The figure shows three views and two pictorial views of one solid part (mm, origin at its lowest corner). Answer the questions. A direction names the side the tool comes from. Coordinates: 2 decimals unless noted, no trailing zeros. Order: outer loops, then holes, each group sorted by start corner. A loop starts at its lowest first (then second) coordinate and runs counter-clockwise, first axis right, second up. Notation, with made-up numbers: (10.5, 67.25) - (53.5, 67.25) arc R29 cw to (53.5, 91.25) - close; hole circle Ø11 at (-6, 21.25). An arc over 180 degrees is marked (long way). Use one line per item in the form item = value.
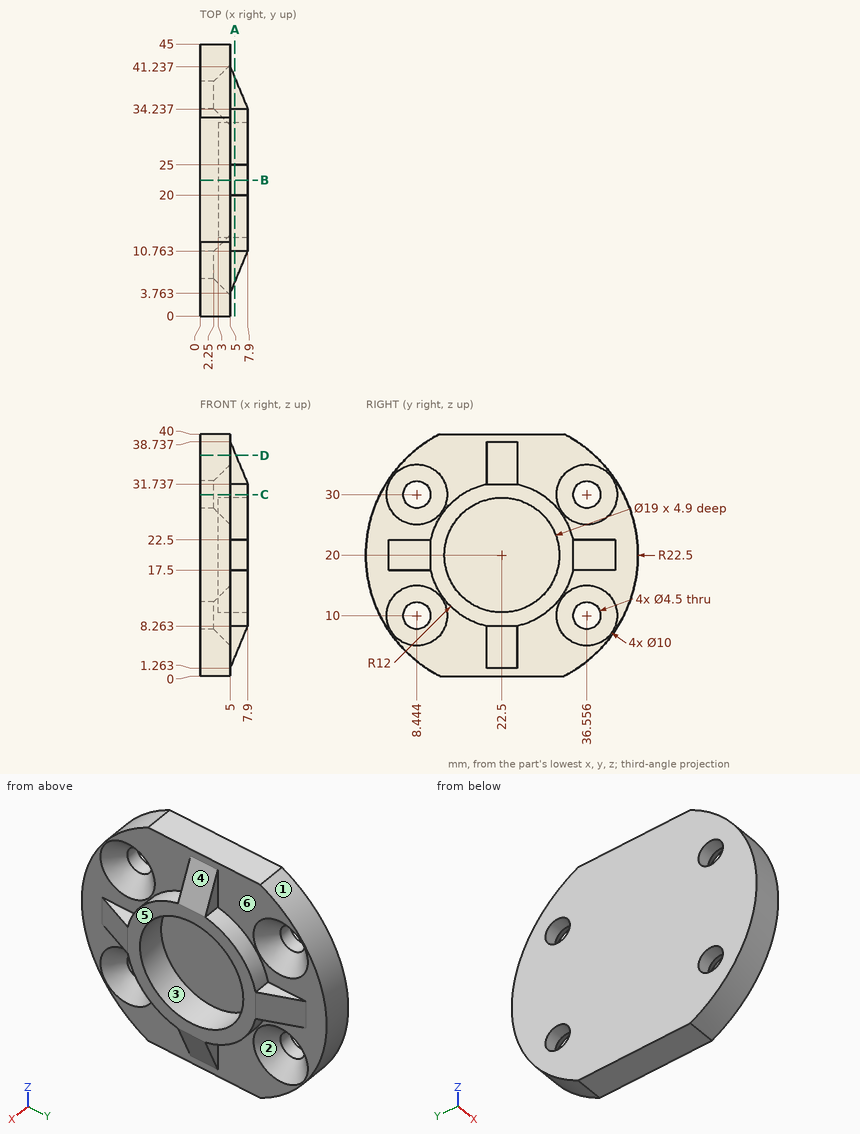
(1) The mould has two halves that part along Y. Classify the marked faces 1, 2, 3 and 4: +Y half, -Y half, draft (parallel to the pull), parting line (faces both ways), or undercut.
Answer list:
face_1 = +Y half
face_2 = undercut
face_3 = undercut
face_4 = draft
(2) Section A-A, the plane x = 5.75 is taken. Write down the section's boundary in (y, z), then the cut area to 3 significant figures.
Answer list:
outline = (5.57, 17.5) - (10.76, 17.5) arc R12 ccw to (20, 8.26) - (20, 3.07) - (25, 3.07) - (25, 8.26) arc R12 ccw to (34.24, 17.5) - (39.43, 17.5) - (39.43, 22.5) - (34.24, 22.5) arc R12 ccw to (25, 31.74) - (25, 36.93) - (20, 36.93) - (20, 31.74) arc R12 ccw to (10.76, 22.5) - (5.57, 22.5) - close; hole circle Ø19 at (22.5, 20)
area = 269 mm2
(3) Section D-D, the plane z = 36.5 is taken. Write down the section's boundary in (x, y).
Answer list:
outline = (0, 7.2) - (5, 7.2) - (5, 20) - (5.93, 20) - (5.93, 25) - (5, 25) - (5, 37.8) - (0, 37.8) - close
(4) Given pin 1 Ø6 at (y, z) = (8.44, 30) entering from +X (1 decimal); pin 2 Ø1.5 at (x, z) = (5.5, 18) entering from +Y; pin 3 Ø0.9 at (x, z) = (6, 5.5) entering from -Y, each flat-ended and moving along its own axis, determine where each tip first touches the part or whether it passes through.
Answer list:
pin_1 = 3
pin_2 = 44.95
pin_3 = 20
(5) Section C-C, the plane z = 30 is taken. Write down the section's boundary in (x, y).
Answer list:
outline = (0, 2.34) - (5, 2.34) - (5, 3.44) - (2.25, 6.19) - (0, 6.19) - close; (0, 10.69) - (2.25, 10.69) - (5, 13.44) - (5, 15.87) - (7.9, 15.87) - (7.9, 29.13) - (5, 29.13) - (5, 31.56) - (2.25, 34.31) - (0, 34.31) - close; (0, 38.81) - (2.25, 38.81) - (5, 41.56) - (5, 42.66) - (0, 42.66) - close
(6) Which of the six approach directions +Z, -Z, +X, -X, +Y, -Y give full straight-line access (tool end or side, diameter ignored) to the marked faces 5 and 6?
Answer list:
face_5 = +Z, -Z, +X, +Y, -Y
face_6 = +X
(7) Straight lines are drawn through the part: L1, parallel to Z at x = 4.5, y = 22.5; L2, parallel to Y at x = 1.8, z = 10 (1 decimal); L3, parallel to Y at x = 6, z = 13.5. For each, find the intervals that lie inside material, in ascending order.
Answer list:
L1 = 0 to 10.5, 29.5 to 40
L2 = 2.3 to 6.2, 10.7 to 34.3, 38.8 to 42.7
L3 = 12.41 to 15.57, 29.43 to 32.59
(8) Section B-B, the plane y = 22.5 is taken. Write down the section's boundary in (x, z), then the cut area to 3 significant figures.
Answer list:
outline = (0, 0) - (5, 0) - (5, 1.26) - (7.9, 8.26) - (7.9, 10.5) - (3, 10.5) - (3, 29.5) - (7.9, 29.5) - (7.9, 31.74) - (5, 38.74) - (5, 40) - (0, 40) - close
area = 195 mm2
